Part model, mm, in its own coordinate system. A direction names the side the tool comes from. Coordinates: 2 decimals unless noted, no trailing zeros. Order: outer loops, then holes, each group sorted by start corner. A loop starts at its lowest first (then second) coordinate and runs counter-clockwise, first axis right, second up.
1) Tool access for faces 4 (the flat face through (58, 11, 0)), 5 (the flat face through (55, 14, 2.5)), 6 (the flat face through (59.692, -14.947, -30.516)), 7 (the flat face through (9.595, -15, -36)): list every direction of +Z, -Z, +X, -X, +Y, -Y with a clear straight run to the whole face (end or side of a thin tool).
2) Mould opens along Y. For faces 1 (the cylindrical face through (7.305, 93.987, 1.521)), 2 (the flat face through (54, 2, 5)), 3 (the flat face through (59.692, -19.024, -40.333)) say: +Y half, -Y half, draft (parallel to the pull), parting line (faces both ways), or undercut.
3) Cut at A-A (y = 50.5). List the corners of the cut face in (x, z).
4) Cut at B-B (x = 23). Give the number of separate pieces and of enclosed holes in the cut face, and give its area (3 significant figures).
5) Wall check: L1, parallel to X at y = 92.5, z = 1.9; L2, parallel to Y at x = 7.5, z = 1.35; L3, parallel to Y at x = 7.5, z = 1.6. Give the ranges that are in metal, low to high.
6) Pin check, flat tips, straight feed: pin 1 Ø7.5 at (y, z) = (-15, -33) entering from -X; pin 2 Ø8 at (x, z) = (66, -27.5) entering from +Y; pin 3 Ø4 at (x, y) = (110.5, 92.5) entering from -Z. Stop position of each tip, or through.
Autodesk Inventor part; units mm, degrees
ref_plane "YZ Plane" through (0, 0, 0) normal (1, 0, 0) x (0, 1, 0)
ref_plane "XZ Plane" through (0, 0, 0) normal (0, 1, 0) x (-1, 0, 0)
ref_plane "XY Plane" through (0, 0, 0) normal (0, 0, 1) x (1, 0, 0)
sketch "Sketch1" plane through (0, 0, 0) normal (0, 0, 1) x (1, 0, 0)
  line L0 (0, 0) -> (118, 0)
  line L1 (118, 0) -> (118, 100)
  line L2 (118, 100) -> (0, 100)
  line L3 (0, 100) -> (0, 0)
  line L4 (-23.6, 0) -> (141.6, 0)
  line L5 (0, -20) -> (0, 120)
  dimension "d3" = 118
  dimension "d4" = 100
  dimension "d45" = 0
  dimension "d46" = 0
extrude "Extrusion1" add sketch "Sketch1" along normal blind 5
sketch "Sketch2" plane through (0, 0, 5) normal (0, 0, 1) x (1, 0, 0)
  line L0 (7, 96) -> (111, 96)
  line L1 (114, 93) -> (114, 7)
  line L2 (111, 4) -> (7, 4)
  line L3 (4, 7) -> (4, 93)
  line L4 (118, 100) -> (0, 100)
  line L5 (0, 100) -> (0, 0)
  line L6 (0, 0) -> (118, 0)
  arc A0 (7, 96) -> (4, 93) centre (7, 93) ccw
  arc A1 (114, 93) -> (111, 96) centre (111, 93) ccw
  arc A2 (111, 4) -> (114, 7) centre (111, 7) ccw
  arc A3 (4, 7) -> (7, 4) centre (7, 7) ccw
  point P0 (4, 96)
  point P1 (114, 4)
  point P2 (114, 96)
  dimension "d7" = 110
  dimension "d8" = 92
  dimension "d10" = 4
  dimension "d11" = 4
  dimension "d12" = 3
extrude "Extrusion2" cut sketch "Sketch2" against normal blind 2
sketch "Sketch3" plane through (0, 0, 3) normal (0, 0, 1) x (1, 0, 0)
  line L0 (12, 12) -> (106, 12)
  line L1 (106, 12) -> (106, 88)
  line L2 (106, 88) -> (12, 88)
  line L3 (12, 88) -> (12, 12)
  line L4 (7, 96) -> (111, 96)
  line L5 (111, 4) -> (7, 4)
  line L6 (4, 7) -> (4, 93)
  line L7 (114, 93) -> (114, 7)
  point P0 (0, 0)
  point P1 (114, 7)
  point P2 (11.024, 100)
  point P3 (121.024, 100)
  point P4 (120, 96)
  point P5 (120, 4)
  dimension "d19" = 8
  dimension "d20" = 8
  dimension "d21" = 8
  dimension "d22" = 8
extrude "Extrusion3" cut sketch "Sketch3" against normal blind 0.5
sketch "Sketch4" plane through (0, 0, 2.5) normal (0, 0, 1) x (1, 0, 0)
  line L0 (15, 85) -> (103, 85)
  line L1 (103, 85) -> (103, 15)
  line L2 (103, 15) -> (15, 15)
  line L3 (15, 15) -> (15, 85)
  line L4 (106, 12) -> (12, 12)
  line L5 (12, 12) -> (12, 88)
  point P0 (0, 0)
  dimension "d25" = 88
  dimension "d26" = 70
  dimension "d27" = 3
  dimension "d28" = 3
extrude "Extrusion4" cut sketch "Sketch4" against normal through all
sketch "Sketch5" plane through (0, 0, 3) normal (0, 0, 1) x (1, 0, 0)
  circle A0 centre (7.5, 7.5) radius 1.5
  circle A1 centre (110.5, 7.5) radius 1.5
  circle A2 centre (110.5, 92.5) radius 1.5
  circle A3 centre (7.5, 92.5) radius 1.5
  line L0 (7, 96) -> (111, 96)
  line L1 (4, 7) -> (4, 93)
  line L2 (111, 4) -> (7, 4)
  line L3 (114, 93) -> (114, 7)
  point P0 (0, 0)
  point P1 (114, 7)
  point P2 (11.024, 100)
  point P3 (121.024, 100)
  point P4 (120, 96)
  point P5 (120, 4)
  dimension "d31" = 3.5
  dimension "d32" = 3.5
  dimension "d33" = 3.5
  dimension "d34" = 3.5
  dimension "d35" = 3.5
  dimension "d36" = 3.5
  dimension "d37" = 3.5
  dimension "d38" = 3.5
  dimension "d39" = 3
  dimension "d40" = 3
  dimension "d41" = 3
  dimension "d42" = 3
extrude "Extrusion5" cut sketch "Sketch5" against normal blind 3.5
sketch "Sketch6" plane through (0, 0, 0) normal (-1, 0, 0) x (0, 0, 1)
  line L0 (-1, 1) -> (-13.2791, -20.2679)
  line L1 (5, 0) -> (5, 100)
  line L2 (1.259, -2.0155) -> (-10.2791, -22)
  line L3 (-13.2791, -20.2679) -> (-10.2791, -22)
  line L4 (-1, 1) -> (0, 1)
  line L5 (0, 0) -> (0, 100)
  line L6 (5, 0) -> (4.5, -0.866)
  line L7 (4.5, -0.866) -> (3.25, -0.866)
  line L8 (3.25, -0.866) -> (1.259, -2.0155)
  line L9 (0, 0) -> (5, 0)
  line L10 (5, 0) -> (0, 0)
  dimension "d47" = 30
  dimension "d48" = 30
  dimension "d49" = 90
  dimension "d50" = 22
  dimension "d51" = 120
  dimension "d52" = 1
  dimension "d53" = 1.25
  dimension "d54" = 150
  dimension "d55" = 0
  dimension "d57" = 90
  dimension "d58" = 1
  dimension "d59" = 3
  dimension "d60" = 1
  dimension "d67" = 30
  dimension "d68" = 120
  dimension "d69" = 150
extrude "Extrusion6" add sketch "Sketch6" against normal blind 118
sketch "Sketch7" plane through (0, -22, -10.2791) normal (0, -0.5, 0.8660254) x (1, 0, 0)
  line L0 (0, 26.6921) -> (118, 26.6921)
  circle A0 centre (25, 13.0581) radius 8
  line L1 (118, 25.0581) -> (0, 25.0581)
  line L2 (0, 0) -> (0, 23.0761)
  point P0 (0, 24.1921)
  dimension "d70" = 16
  dimension "d71" = 12
  dimension "d72" = 25
extrude "Extrusion7" cut sketch "Sketch7" against normal up to next
sketch "Sketch8" plane through (0, -22, -10.2791) normal (0, -0.5, 0.8660254) x (1, 0, 0)
  circle A0 centre (25, 13.0581) radius 8
  circle A1 centre (25, 13.0581) radius 11.125
  point P0 (0, 24.1921)
  dimension "d75" = 22.25
extrude "Extrusion8" cut sketch "Sketch8" along normal blind 1
sketch "Sketch9" plane through (0, 100, 0) normal (-1, 0, 0) x (0, 0, 1)
  line L0 (-10.2791, -122) -> (1.259, -102.0155)
  line L1 (-10.2791, -122) -> (-11.7791, -124.5981)
  line L2 (-11.7791, -124.5981) -> (-32.7791, -112.4737)
  line L3 (-32.7791, -112.4737) -> (-31.2791, -109.8756)
  line L4 (-1, -99) -> (-13.2791, -120.2679)
  line L5 (-31.2791, -109.8756) -> (-13.2791, -120.2679)
  line L6 (-13.2791, -120.2679) -> (-10.2791, -122)
  point P0 (0, -100)
  dimension "d79" = 3
  dimension "d80" = 90
  dimension "d82" = 90
  dimension "d83" = 90
  dimension "d84" = 90
  dimension "d85" = 21
extrude "Extrusion9" add sketch "Sketch9" against normal blind 118
sketch "Sketch10" plane through (118, 100, 0) normal (1, 0, 0) x (0, 0, -1)
  line L0 (35.9184, -109.7111) -> (41.7463, -118.0342)
  line L1 (31.2791, -109.8756) -> (32.7791, -112.4737)
  line L2 (41.7463, -118.0342) -> (38.8793, -120.0417)
  line L3 (32.7791, -112.4737) -> (33.3495, -112.1444)
  line L4 (38.8793, -120.0417) -> (33.3495, -112.1444)
  line L5 (31.2791, -109.8756) -> (34.6648, -107.9209)
  line L6 (41.7463, -118.0342) -> (34.6648, -107.9209)
  line L7 (32.7791, -112.4737) -> (11.7791, -124.5981)
  point P0 (0, -100)
  dimension "d88" = 3.5
  dimension "d93" = 3.5
  dimension "d97" = 0
extrude "Extrusion10" add sketch "Sketch10" against normal blind 118
fillet "Fillet1" radius 8 1 edges at (59, 1, 0)
chamfer "Chamfer1" distance 2.2 angle 45 1 edges at (59, -7.9209, -34.6648)
chamfer "Chamfer2" distance 2 distance2 8 1 edges at (59, -12.1444, -33.3495) measured on face at (78.6667, -14.7768, -35.1927)
sketch "Sketch11" plane through (25, -10.6913, -3.75) normal (0, -0.5, 0.8660254) x (1, 0, 0)
  line L0 (-25, -16.0581) -> (-25, 10.0179)
  line L1 (-25, 10.0179) -> (-25, 4.5179)
  line L2 (-25, 4.5179) -> (-15.4052, -16.0581)
  line L3 (-25, -25.6623) -> (-25, -18.0505)
  line L4 (-25, 4.5179) -> (-25, -25.6623)
  line L5 (-25, -25.6623) -> (-15.4052, -25.6623)
  line L6 (-25, -16.0581) -> (93, -16.0581)
  line L7 (-15.4052, -16.0581) -> (-15.4052, -25.6623)
  line L8 (93, 10.0179) -> (93, 4.5179)
  line L9 (93, 4.5179) -> (83.4052, -16.0581)
  line L10 (83.4052, -16.0581) -> (83.4052, -25.6623)
  line L11 (93, -25.6623) -> (83.4052, -25.6623)
  line L12 (93, -25.6623) -> (93, 4.5179)
  line L13 (93, 10.0179) -> (93, -16.0581)
  point P0 (-25, 11.134)
  point P1 (-25, -18.0505)
  dimension "d101" = 5.5
  dimension "d102" = 25
  dimension "d105" = 5.5
  dimension "d106" = 0
  dimension "d107" = 35.6803
extrude "Extrusion11" cut sketch "Sketch11" against normal through all
equation "\"d39\" = d41"
equation "\"d40\" = d41"
equation "\"d42\" = d41"
properties part number "MainHousing_FrontMainShell"
Geometry check:
1. face 4: -Z, +X, -X, +Y
1. face 5: +Z
1. face 6: +X, -X, -Y
1. face 7: -Z, -X, -Y
2. face 1: undercut
2. face 2: draft
2. face 3: -Y half
3. outline: (0, 0) - (15, 0) - (15, 2.5) - (12, 2.5) - (12, 3) - (4, 3) - (4, 5) - (0, 5) - close; (103, 0) - (118, 0) - (118, 5) - (114, 5) - (114, 3) - (106, 3) - (106, 2.5) - (103, 2.5) - close
4. separate pieces: 3
4. enclosed holes: 0
4. area: 263 mm2
5. L1: x = 0 to 6, 9 to 109, 112 to 118
5. L2: y = -1.96 to 6, 9 to 91, 94 to 100
5. L3: y = -1.82 to 6, 9 to 91, 94 to 100
6. pin 1: stops at x = 8.92
6. pin 2: stops at y = -9.75
6. pin 3: stops at z = 0
